from build123d import *

# Parameters (mm, degrees)
F0_W     = 4.490128
F0_H     = 4.490128
F1_DEPTH = 3.41884


with BuildPart() as f1:
    # F0 (on Top) → F1 (new body)
    with BuildSketch(Plane.XY):
        with BuildLine():
            Line((5.55625, 0), (5.55625, 38.1))
            ThreePointArc((5.55625, 38.1), (3.928862, 42.028862), (0, 43.65625))
            Line((0, 43.65625), (-38.1, 43.65625))
            ThreePointArc((-38.1, 43.65625), (-43.233306, 40.226285), (-42.028862, 34.171138))
            Line((-42.028862, 34.171138), (-3.928862, -3.928862))
            ThreePointArc((-3.928862, -3.928862), (2.126285, -5.133306), (5.55625, 0))
        make_face()
        Rectangle(F0_W, F0_H, mode=Mode.SUBTRACT)
        with Locations((-38.1, 38.1)):
            Rectangle(F0_W, F0_H, mode=Mode.SUBTRACT)
        with Locations((0, 38.1)):
            Rectangle(F0_W, F0_H, mode=Mode.SUBTRACT)
    extrude(amount=F1_DEPTH)


solid = f1.part
Could you check a few things on this model? Use its own coordinates, in mm. A direction names the side the tool comes from. Coordinates: 2 decimals unless noted, no trailing zeros. Order: outer loops, then holes, each group sorted by start corner. A loop starts at its lowest first (then second) coordinate and runs counter-clockwise, first axis right, second up. Notation, with made-up numbers: (14, 42) -> (43, 42) arc R12 cw to (43, 49) -> close; hole circle Ø7 at (51, -34.75). An arc over 180 degrees is marked (long way). One line per question, with ' | ' between items.
Q1. Imagine slicing it at D-D on x = -8. Please give me the cut outline in (y, z).
Return value:
outline: (0.14, 0) -> (43.66, 0) -> (43.66, 3.42) -> (0.14, 3.42) -> close
Q2. Imagine slicing it at C-C on y = 33. Please give me the cut outline in (x, z).
Return value:
outline: (-40.86, 0) -> (5.56, 0) -> (5.56, 3.42) -> (-40.86, 3.42) -> close
Q3. If I drill on L1, parallel to X at y = 37.5, z = 2.55; L2, parallel to Y at x = -37, z = 2.9; L3, parallel to X at y = 0, z = 1.85, over which ranges is the centre line in solid material (lowest first)?
Return value:
L1: -43.62 to -40.35, -35.85 to -2.25, 2.25 to 5.56 | L2: 29.14 to 35.85, 40.35 to 43.66 | L3: -7.86 to -2.25, 2.25 to 5.56
Q4. Imagine slicing it at A-A on z = 1.25. Please give me the cut outline in (x, y).
Return value:
outline: (-42.03, 34.17) -> (-3.93, -3.93) arc R5.56 ccw to (5.56, 0) -> (5.56, 38.1) arc R5.56 ccw to (0, 43.66) -> (-38.1, 43.66) arc R5.56 ccw to start; hole (-40.35, 35.85) -> (-35.85, 35.85) -> (-35.85, 40.35) -> (-40.35, 40.35) -> close; hole (-2.25, -2.25) -> (2.25, -2.25) -> (2.25, 2.25) -> (-2.25, 2.25) -> close; hole (-2.25, 35.85) -> (2.25, 35.85) -> (2.25, 40.35) -> (-2.25, 40.35) -> close
Q5. Thinking about a two-plate mould opening in X: for faces 3 (the face through (-23.25, 15.39, 1.69)), 4 (the face through (-14, 25, 0)), 5 (the face through (-38, 40.345, 2)), which applies, pulls with the +X half, pulls with the -X half, needs draft (parallel to the pull), parting line crosses it, or undercut?
Return value:
face 3: pulls with the -X half | face 4: needs draft | face 5: undercut
Q6. On a 3-axis mill with a long thin cutter (end or side, diameter ignored), from which of +Z, -Z, +X, -X, +Y, -Y can I reach the whole of each face in a straight line? I mean faces 1 (the face through (-19, 43.656, 2)), 2 (the face through (-2.245, 38, 2)). Say none if no direction works.
Return value:
face 1: +Z, -Z, +X, -X, +Y | face 2: +Z, -Z
Q7. Imagine slicing it at B-B on x = -36.5. Please give me the cut outline in (y, z).
Return value:
outline: (28.64, 0) -> (35.85, 0) -> (35.85, 3.42) -> (28.64, 3.42) -> close; (40.35, 0) -> (43.66, 0) -> (43.66, 3.42) -> (40.35, 3.42) -> close
Q8. I'm going to push flat-ended pins straight in: P1, Ø2, axis at x = -8.5, z = 3, coming from the -Y side; P2, Ø12, axis at x = -24, y = 6.5, coming from the -Z side. Where does each tip first touch, or does it pass through?
Return value:
P1: y = -0.36 | P2: through
